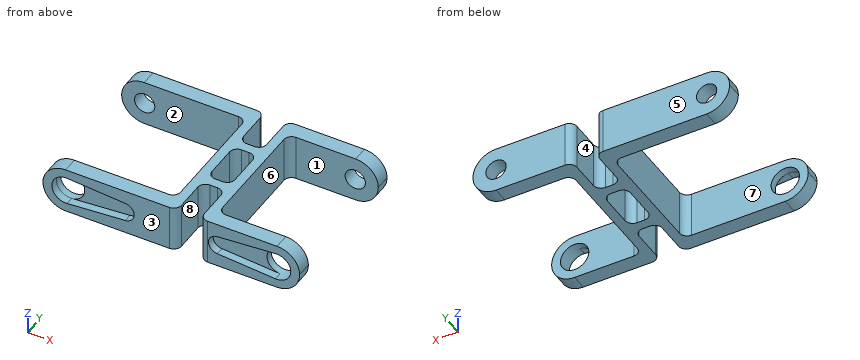
from build123d import *

# Parameters (mm, degrees)
PAD_DEPTH       = 12
SKETCH001_R     = 3.7
POCKET_DEPTH    = 5
POCKET001_DEPTH = 2.1
SKETCH003_R     = 2.65
POCKET002_DEPTH = 5
FILLET_R        = 6
FILLET001_R     = 6
FILLET002_R     = 6
FILLET003_R     = 6
FILLET004_R     = 5.9
FILLET005_R     = 5.9
FILLET006_R     = 5.9
FILLET007_R     = 5.9


with BuildPart() as part:
    # Sketch → Pad (new body)
    with BuildSketch(Plane.XY):
        with BuildLine():
            Line((-3, 10.5), (-3, 18))
            ThreePointArc((-3, 18), (-3.585786, 19.414214), (-5, 20))
            Line((-5, 20), (-38, 20))
            Line((-38, 20), (-38, 16))
            Line((-38, 16), (-7.5, 16))
            ThreePointArc((-5.5, 14), (-6.085786, 15.414214), (-7.5, 16))
            Line((-5.5, 14), (-5.5, -14))
            ThreePointArc((-7.5, -16), (-6.085786, -15.414214), (-5.5, -14))
            Line((-7.5, -16), (-38, -16))
            Line((-38, -16), (-38, -20))
            Line((-38, -20), (-5, -20))
            ThreePointArc((-5, -20), (-3.585786, -19.414214), (-3, -18))
            Line((-3, -18), (-3, -10.5))
            ThreePointArc((-1, -8.5), (-2.414214, -9.085786), (-3, -10.5))
            Line((-1, -8.5), (1, -8.5))
            ThreePointArc((3, -10.5), (2.414214, -9.085786), (1, -8.5))
            Line((3, -10.5), (3, -18))
            ThreePointArc((3, -18), (3.585786, -19.414214), (5, -20))
            Line((5, -20), (29, -20))
            Line((29, -20), (29, -16))
            Line((29, -16), (7.5, -16))
            ThreePointArc((5.5, -14), (6.085786, -15.414214), (7.5, -16))
            Line((5.5, -14), (5.5, 14))
            ThreePointArc((7.5, 16), (6.085786, 15.414214), (5.5, 14))
            Line((7.5, 16), (29, 16))
            Line((29, 16), (29, 20))
            Line((29, 20), (5, 20))
            ThreePointArc((5, 20), (3.585786, 19.414214), (3, 18))
            Line((3, 18), (3, 10.5))
            ThreePointArc((1, 8.5), (2.414214, 9.085786), (3, 10.5))
            Line((1, 8.5), (-1, 8.5))
            ThreePointArc((-3, 10.5), (-2.414214, 9.085786), (-1, 8.5))
        make_face()
        with BuildLine():
            Line((3, -4), (3, 4))
            ThreePointArc((3, 4), (2.414214, 5.414214), (1, 6))
            Line((1, 6), (-1, 6))
            ThreePointArc((-1, 6), (-2.414214, 5.414214), (-3, 4))
            Line((-3, 4), (-3, -4))
            ThreePointArc((-3, -4), (-2.414214, -5.414214), (-1, -6))
            Line((-1, -6), (1, -6))
            ThreePointArc((1, -6), (2.414214, -5.414214), (3, -4))
        make_face(mode=Mode.SUBTRACT)
    extrude(amount=PAD_DEPTH)

    # Sketch001 (on Face11 of Pad) → Pocket (cut)
    with BuildSketch(Plane.XZ.offset(20)):
        with Locations((-32, 6)):
            Circle(SKETCH001_R)
        with Locations((23, 6)):
            Circle(SKETCH001_R)
    extrude(amount=-POCKET_DEPTH, mode=Mode.SUBTRACT)

    # Sketch002 (on Face23 of Pocket) → Pocket001 (cut)
    with BuildSketch(Plane.XZ.offset(20)):
        with BuildLine():
            ThreePointArc((-31.709804, 9.688602), (-35.7, 6), (-31.709804, 2.311398))
            Line((-31.709804, 2.311398), (-16.503922, 3.507701))
            ThreePointArc((-16.503922, 3.507701), (-14.2, 6), (-16.503922, 8.492299))
            Line((-16.503922, 8.492299), (-31.709804, 9.688602))
        make_face()
        with BuildLine():
            ThreePointArc((22.709804, 2.311398), (26.7, 6), (22.709804, 9.688602))
            Line((22.709804, 9.688602), (7.503922, 8.492299))
            ThreePointArc((7.503922, 8.492299), (5.2, 6), (7.503922, 3.507701))
            Line((7.503922, 3.507701), (22.709804, 2.311398))
        make_face()
    extrude(amount=-POCKET001_DEPTH, mode=Mode.SUBTRACT)

    # Sketch003 (on Face31 of Pocket001) → Pocket002 (cut)
    with BuildSketch(Plane(origin=(0, 20, 0), x_dir=(-1, 0, 0), z_dir=(0, 1, 0))):
        with Locations((-23, 6)):
            Circle(SKETCH003_R)
        with Locations((32, 6)):
            Circle(SKETCH003_R)
    extrude(amount=-POCKET002_DEPTH, mode=Mode.SUBTRACT)

    # Fillet
    fillet_edges = [part.edges().sort_by_distance(p)[0] for p in [
        (29, 18, 0),
    ]]
    fillet(fillet_edges, radius=FILLET_R)

    # Fillet001
    fillet001_edges = [part.edges().sort_by_distance(p)[0] for p in [
        (29, -18, 0),
    ]]
    fillet(fillet001_edges, radius=FILLET001_R)

    # Fillet002
    fillet002_edges = [part.edges().sort_by_distance(p)[0] for p in [
        (-38, -18, 0),
    ]]
    fillet(fillet002_edges, radius=FILLET002_R)

    # Fillet003
    fillet003_edges = [part.edges().sort_by_distance(p)[0] for p in [
        (-38, 18, 0),
    ]]
    fillet(fillet003_edges, radius=FILLET003_R)

    # Fillet004
    fillet004_edges = [part.edges().sort_by_distance(p)[0] for p in [
        (29, -18, 12),
    ]]
    fillet(fillet004_edges, radius=FILLET004_R)

    # Fillet005
    fillet005_edges = [part.edges().sort_by_distance(p)[0] for p in [
        (29, 18, 12),
    ]]
    fillet(fillet005_edges, radius=FILLET005_R)

    # Fillet006
    fillet006_edges = [part.edges().sort_by_distance(p)[0] for p in [
        (-38, 18, 12),
    ]]
    fillet(fillet006_edges, radius=FILLET006_R)

    # Fillet007
    fillet007_edges = [part.edges().sort_by_distance(p)[0] for p in [
        (-38, -18, 12),
    ]]
    fillet(fillet007_edges, radius=FILLET007_R)


solid = part.part
For this review, take the finished solid that the model builds, in its own axes (mm). Face numbers are marked on the shaded views. A direction names the side the tool comes from. Round coordinates to 2 decimals unless told otherwise and drop trailing zeros. Loops run counter-clockwise (first coordinate to the right, second up) from the corner with the lowest first, then second, coordinate; pieces in that order, holes last. Notation, with made-up numbers: (-14, 87) - (42, 87) arc R17 ccw to (42, 106) - close; hole circle Ø6 at (15, -17). An arc over 180 degrees is marked (long way). Answer as CSV lines item,"result".
(1) Insertion check: P1, Ø4, axis at y = -14.5, z = 7.5, coming from the -X side; P2, Ø2, axis at x = -0.5, z = 6, coming from the +Y side; P3, Ø4, axis at y = -6, z = 4.5, coming from the -X side; P4, Ø1, axis at x = 0.5, z = 3.5, coming from the +Y side. Each pin has a flat end and moves straight along its axis. Give the tip position at first contact, or say it passes through.
Checked values:
P1,"stops at x = -38"
P2,"stops at y = 8.56"
P3,"stops at x = -5.5"
P4,"stops at y = 8.5"
(2) Wall thickness on line 1 (Y direction, x = 14, z = 8.5); line 2 (Z direction, x = 23, y = 19); line 3 (Z direction, x = -32, y = -16.45): over which ranges is each line inside the solid? List them lowest first.
Checked values:
line 1,"y = -17.9 to -16, 16 to 20"
line 2,"z = 0 to 3.35, 8.65 to 12"
line 3,"z = 0 to 2.3, 9.7 to 12"
(3) Consider section C-C on x = 22. Give the boundary of the cut face in (y, z), then the cut area to 3 significant figures.
Checked values:
outline,"(-20, 0) - (-16, 0) - (-16, 2.44) - (-17.9, 2.44) - (-17.9, 2.37) - (-20, 2.37) - close; (-20, 9.63) - (-17.9, 9.63) - (-17.9, 9.56) - (-16, 9.56) - (-16, 12) - (-20, 12) - close; (16, 0) - (20, 0) - (20, 3.55) - (16, 3.55) - close; (16, 8.45) - (20, 8.45) - (20, 12) - (16, 12) - close"
area,"47.6 mm2"
(4) Mouldability with a two-part tool opening along Y and no side actions: class the marked faces 5, 6, 7 and 8 as +Y half, -Y half, draft (parallel to the pull), parting line (faces both ways), or undercut.
Checked values:
face 5,"+Y half"
face 6,"undercut"
face 7,"undercut"
face 8,"draft"
(5) Consider section B-B on x = -9. Give the boundary of the cut face in (y, z).
Checked values:
outline,"(-20, 0) - (-16, 0) - (-16, 12) - (-20, 12) - close; (16, 0) - (20, 0) - (20, 12) - (16, 12) - close"
(6) Tool access review of the marked faces 1, 2, 3 and 4: name each direction out of +Z, -Z, +X, -X, +Y, -Y from which nothing blocks a thin tool from reaching the whole face with its end or side.
Checked values:
face 1,"+Z, -Z, +X"
face 2,"+Z, -Z, -X"
face 3,"+Z, -Z, +X, -X, -Y"
face 4,"+Z, -Z, +Y"
(7) Consider section D-D on y = 7. Give the boundary of the cut face in (x, z), then the cut area to 3 significant figures.
Checked values:
outline,"(-5.5, 0) - (5.5, 0) - (5.5, 12) - (-5.5, 12) - close"
area,"132 mm2"
(8) Consider section A-A on y = 17. Give the boundary of the cut face in (x, z).
Checked values:
outline,"(-38, 6) arc R6 ccw to (-32, 0) - (-3, 0) - (-3, 12) - (-32.1, 12) arc R5.9 ccw to (-38, 6.1) - close; (3, 0) - (23, 0) arc R6 ccw to (29, 6) - (29, 6.1) arc R5.9 ccw to (23.1, 12) - (3, 12) - close; hole circle Ø5.3 at (-32, 6); hole circle Ø5.3 at (23, 6)"
